from build123d import *

# Parameters (mm, degrees)
F0_W     = 154
F0_H     = 40
F1_DEPTH = 32.5
F2_T     = -6
F4_DEPTH = 7


with BuildPart() as f1:
    # F0 (on Front) → F1 (new body, symmetric)
    with BuildSketch(Plane.XZ):
        Rectangle(F0_W, F0_H)
    extrude(amount=F1_DEPTH, both=True)

    # F2
    f2_openings = [f1.faces().sort_by_distance(p)[0] for p in [
        (0, 0, -20),
        (-77, 0, 0),
        (77, 0, 0),
    ]]
    offset(amount=F2_T, openings=f2_openings)

    # F3 (on face) → F4 (cut)
    with BuildSketch(Plane.XY.offset(20)):
        with BuildLine():
            Line((30, 25), (-30, 25))
            ThreePointArc((-30, 25), (-55, 0), (-30, -25))
            Line((-30, -25), (30, -25))
            ThreePointArc((30, -25), (55, 0), (30, 25))
        make_face()
    extrude(amount=-F4_DEPTH, mode=Mode.SUBTRACT)


solid = f1.part
Verification items for the finished model (mm, model axes). A direction names the side the tool comes from. Coordinates: 2 decimals unless noted, no trailing zeros. Write each loop counter-clockwise with the first axis right and the second up, starting at its lowest first coordinate (ties: lowest second). Pieces come first, ordered by that corner, then holes. Notation, with made-up numbers: M 61.25,-27.75 L 120.25,-27.75 A17 cw 120.25,0.25 Z; hole C 37.5,27.5 d7. An arc over 180 degrees is marked long. One line per question, with ' | ' between items.
1) Material ranges on L1, parallel to Y at x = -56, z = 2; L2, parallel to Z at x = 68.5, y = -3.5; L3, parallel to X at y = 19.5, z = 16.5, recorded low to high.
Solutions:
L1: -32.5 to -26.5, 26.5 to 32.5 | L2: 14 to 20 | L3: -77 to -45.64, 45.64 to 77
2) Sectioned sample at A-A on z = 3. Record the cut outline in (x, y), then the cut area to 3 significant figures.
Solutions:
outline: M -77,-32.5 L 77,-32.5 L 77,-26.5 L -77,-26.5 Z; M -77,26.5 L 77,26.5 L 77,32.5 L -77,32.5 Z | area: 1,850 mm^2
3) Sectioned sample at C-C on x = -58. Record the cut outline in (y, z).
Solutions:
outline: M -32.5,-20 L -26.5,-20 L -26.5,14 L 26.5,14 L 26.5,-20 L 32.5,-20 L 32.5,20 L -32.5,20 Z
4) Release check for a two-part mould opening along Y. For faces 1 (the face through (54.994, -0.55, 17.042)), 2 (the face through (-1, -30, -20)), 3 (the face through (-1, -32.5, 0)), 4 (the face through (0, -26, 14)) record: +Y half, -Y half, draft (parallel to the pull), parting line (faces both ways), or undercut.
Solutions:
face 1: undercut | face 2: draft | face 3: -Y half | face 4: undercut
5) Access from +Z, -Z, +X, -X, +Y, -Y to the whole of each face (thin tool, end or side, straight path). Record for faces 5 (the face through (-1, 26.5, -3)), 6 (the face through (77, -15, 15)), 7 (the face through (0, -25, 17)).
Solutions:
face 5: -Z, +X, -X | face 6: +Z, -Z, +X, +Y, -Y | face 7: +Z, -Z
6) Sectioned sample at B-B on y = 0. Record the cut outline in (x, z).
Solutions:
outline: M -77,14 L -55,14 L -55,20 L -77,20 Z; M 55,14 L 77,14 L 77,20 L 55,20 Z
